Answer from the drawing. Dimensions are ordinates in mm from the lowest x, y and z of the part. A direction names the side the tool comes from. Round coordinates to 2 decimals unless told otherwise and drop trailing zeros. Loops run counter-clockwise (first coordinate to the right, second up) from the corner with the lowest first, then second, coordinate; pieces in that order, holes last. Notation, with made-up numbers: (-19.75, -22) - (-9.75, -22) arc R12 ccw to (-9.75, 0) - close; hole circle Ø9 at (-24.75, 54). An arc over 180 degrees is marked (long way). Answer as CSV lines item,"result". Start each with the question number.
Q1. Straight lines are drawn through the part: L1, parallel to Y at x = 19, z = 0.4; L2, parallel to X at y = 13.5, z = 3.4; L3, parallel to Y at x = 34.5, z = 3.65. For each, find the intervals that lie inside material, in ascending order. Write a range as [from, to].
Q2. Section C-C on x = 69.5 is taken. Write down the section's boundary in (y, z).
Q3. Section A-A on z = 1.3 is taken. Write down the section's boundary in (x, y).
Q4. Section B-B on y = 11.25 is taken. Write down the section's boundary in (x, z), then the cut area to 3 significant figures.
Q5. Each of these flat-tipped pins is pushed along its axis until it touches: pin 1 Ø3 at (y, z) = (11, 2) entering from -X; pin 2 Ø3 at (x, y) = (38, 13.5) entering from -Z; pin 3 Ø2 at (y, z) = (8, 1.5) entering from +X. Where does it stop, or does it pass through?
Q6. Section D-D on x = 4 is taken. Write down the section's boundary in (y, z), then the cut area to 3 significant figures.
Q7. For the marked faces 1, 2 and 3, determine the directions among +Z, -Z, +X, -X, +Y, -Y from which every point of the face is accessible in a straight line to the end or side of a thin tool.
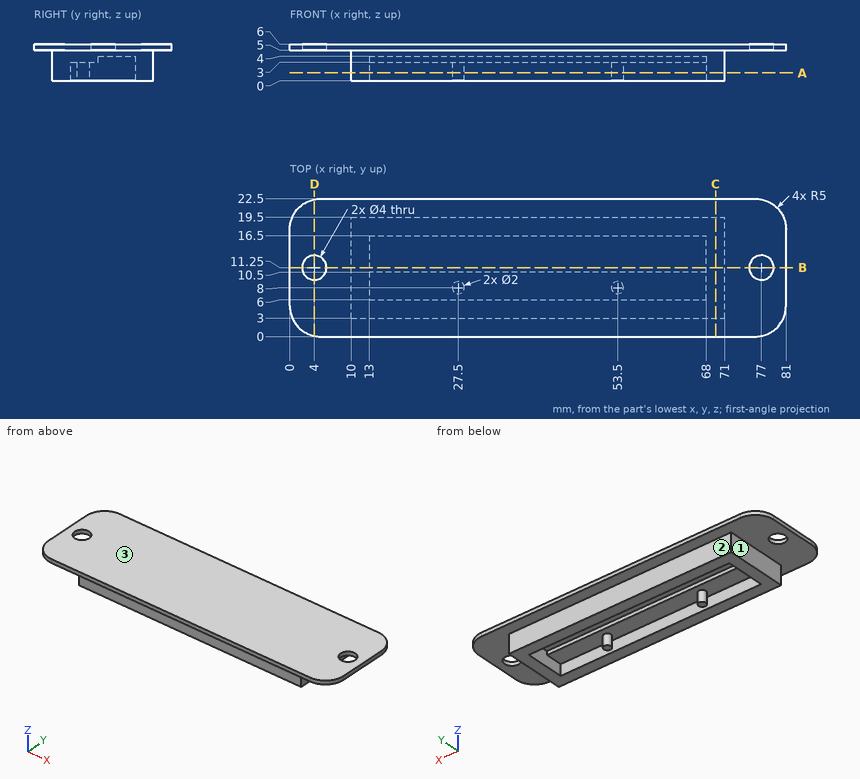
Findings:
1,L1,"y = [3, 6], [16.5, 19.5]"
1,L2,"x = [10, 13], [68, 71]"
1,L3,"y = [3, 10.5], [16.5, 19.5]"
2,outline,"(0, 5) - (3, 5) - (3, 0) - (19.5, 0) - (19.5, 5) - (22.5, 5) - (22.5, 6) - (0, 6) - close"
3,outline,"(10, 3) - (71, 3) - (71, 19.5) - (10, 19.5) - close; circle Ø2 at (27.5, 8); circle Ø2 at (53.5, 8); hole (13, 6) - (68, 6) - (68, 16.5) - (13, 16.5) - close"
4,outline,"(0, 5) - (2, 5) - (2, 6) - (0, 6) - close; (6, 5) - (10, 5) - (10, 0) - (13, 0) - (13, 4) - (68, 4) - (68, 0) - (71, 0) - (71, 5) - (75, 5) - (75, 6) - (6, 6) - close; (79, 5) - (81, 5) - (81, 6) - (79, 6) - close"
4,area,"158 mm^2"
5,pin 1,"stops at x = 10"
5,pin 2,"stops at z = 4"
5,pin 3,"stops at x = 71"
6,outline,"(0.1, 5) - (9.25, 5) - (9.25, 6) - (0.1, 6) - close; (13.25, 5) - (22.4, 5) - (22.4, 6) - (13.25, 6) - close"
6,area,"18.3 mm^2"
7,face 1,"-Z, -X, +Y, -Y"
7,face 2,"-Z, +X, -X, +Y"
7,face 3,"+Z, +X, -X, +Y, -Y"
